Read the model definition and answer for the solid it produces. Units are mm, in the model's axes. A direction names the side the tool comes from. Round coordinates to 2 decimals unless told otherwise and drop trailing zeros. Write each loop counter-clockwise with the first axis right and the second up, starting at its lowest first coordinate (ties: lowest second). Pieces come first, ordered by that corner, then holes. Notation, with made-up numbers: (9, 34) -> (16, 34) arc R22 ccw to (16, 72) -> close; hole circle Ø6 at (17, -26.75). An arc over 180 degrees is marked (long way). Return JSON: item names as keys, results as strings.
from build123d import *

# Parameters (mm, degrees)
F0_W     = 55
F0_H     = 30
F1_DEPTH = 12
F3_D     = 5
F3_DEPTH = 25
F4_W     = 55
F4_H     = 58
F4_H_2   = 12
F5_DEPTH = 12
F7_D     = 12
F7_DEPTH = 12


with BuildPart() as f1:
    # F0 (on Top) → F1 (new body)
    with BuildSketch(Plane.XY):
        Rectangle(F0_W, F0_H)
    extrude(amount=F1_DEPTH)

    # F3
    with Locations(Plane.XY.offset(12)):
        with Locations((-15, 0), (15, 0)):
            Hole(F3_D / 2, depth=F3_DEPTH)

    # F4 (on face) → F5 (join)
    with BuildSketch(Plane.XZ.offset(15)):
        with Locations((0, -29)):
            Rectangle(F4_W, F4_H)
        with Locations((0, 6)):
            Rectangle(F4_W, F4_H_2)
    extrude(amount=F5_DEPTH)

    # F7
    with Locations(Plane(origin=(0, -15, 0), x_dir=(-1, 0, 0), z_dir=(0, 1, 0))):
        with Locations((12.5, -13), (12.5, -43), (-12.5, -43), (-12.5, -13)):
            Hole(F7_D / 2, depth=F7_DEPTH)


solid = f1.part
Item 1: Section A-A (y = 0) is taken. Give the vertices of the cut face in (x, z), then the cut area to 3 significant figures.
Worked answers:
{"outline": "(-27.5, 0) -> (-17.5, 0) -> (-17.5, 12) -> (-27.5, 12) -> close; (-12.5, 0) -> (12.5, 0) -> (12.5, 12) -> (-12.5, 12) -> close; (17.5, 0) -> (27.5, 0) -> (27.5, 12) -> (17.5, 12) -> close", "area": "540 mm2"}
Item 2: For a pull along Y with two mould halves and no side action, classify faces 3 (the cylindrical face through (17.5, 0.1, 5.9)), 4 (the flat face through (0, -27, -23)), 5 (the flat face through (27.5, -20, -16)), 6 (the flat face through (0, 15, 6)) as released by +Y, released by -Y, zero draft, split by the parting line, or undercut.
Worked answers:
{"face 3": "undercut", "face 4": "released by -Y", "face 5": "zero draft", "face 6": "released by +Y"}
Item 3: Flat-ended cylindrical pins translate along their axes: pin 1 (6 mm diameter, centred on x = 15, y = 0, fed in from -Z); pin 2 (16.5 mm diameter, centred on x = 9.5, z = -17, fed in from +Y); pin 3 (10 mm diameter, centred on x = -4.5, z = -2, fed in from +Y). Find the tip coordinate at first contact, or state that the pin passes through.
Worked answers:
{"pin 1": "stops at z = 0", "pin 2": "stops at y = -15", "pin 3": "stops at y = 15"}
Item 4: Section B-B (z = -13) is taken. Give the vertices of the cut face in (x, y), then the cut area to 3 significant figures.
Worked answers:
{"outline": "(-27.5, -27) -> (-18.5, -27) -> (-18.5, -15) -> (-27.5, -15) -> close; (-6.5, -27) -> (6.5, -27) -> (6.5, -15) -> (-6.5, -15) -> close; (18.5, -27) -> (27.5, -27) -> (27.5, -15) -> (18.5, -15) -> close", "area": "372 mm2"}
Item 5: Section C-C (x = -24) is taken. Give the vertices of the cut face in (y, z), then the cut area to 3 significant figures.
Worked answers:
{"outline": "(-27, -58) -> (-15, -58) -> (-15, 0) -> (15, 0) -> (15, 12) -> (-27, 12) -> close", "area": "1,200 mm2"}
Item 6: A tool of negligible diameter and unlimited length cuts with its end or side. For faces 1 (the flat face through (0, -21, -58)), 2 (the flat face through (0, 0, 0)), from which of +Z, -Z, +X, -X, +Y, -Y can it reach the whole face along a straight path? Write none if from no direction.
Worked answers:
{"face 1": "-Z, +X, -X, +Y, -Y", "face 2": "-Z, +X, -X, +Y"}
Item 7: Straight lines are drawn through the part: L1, parallel to Z at x = -12.5, y = -20.75; L2, parallel to Y at x = -15, z = 5; L3, parallel to Z at x = 11, y = -24.5. For each, find the intervals that lie inside material, in ascending order. Write a range as [from, to].
Worked answers:
{"L1": "z = [-58, -49], [-37, -19], [-7, 12]", "L2": "y = [-27, -2.5], [2.5, 15]", "L3": "z = [-58, -48.81], [-37.19, -18.81], [-7.19, 12]"}
Item 8: Section D-D (z = 5.5) is taken. Give the vertices of the cut face in (x, y), then the cut area to 3 significant figures.
Worked answers:
{"outline": "(-27.5, -27) -> (27.5, -27) -> (27.5, 15) -> (-27.5, 15) -> close; hole circle Ø5 at (-15, 0); hole circle Ø5 at (15, 0)", "area": "2,270 mm2"}
